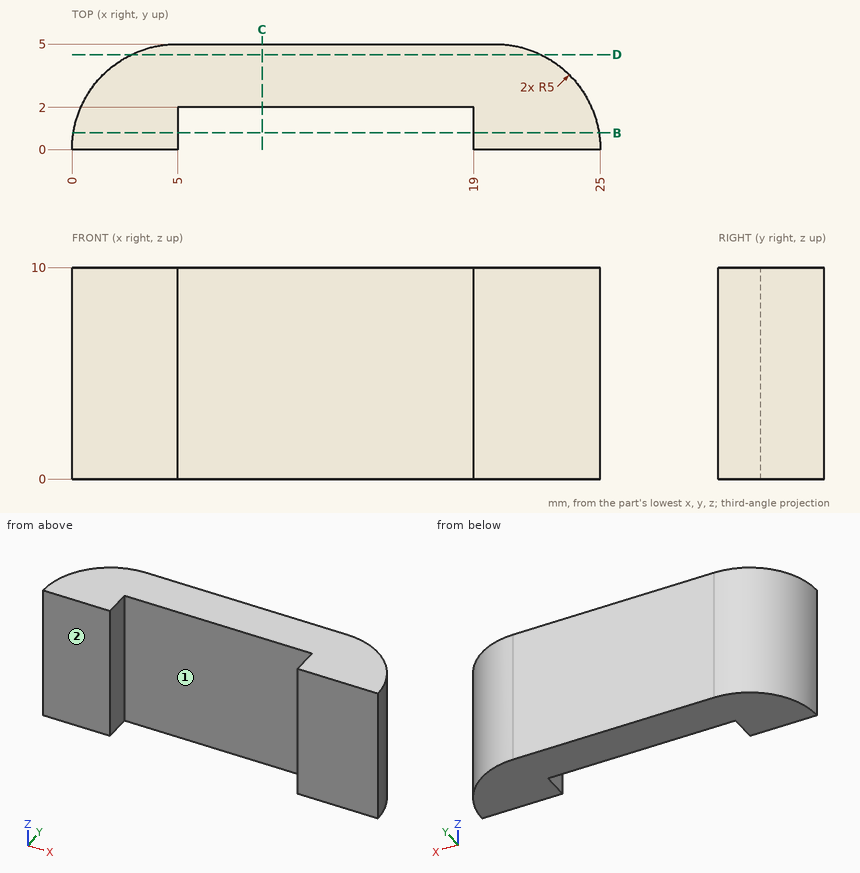
Drawing for the job (mm, zero at the part's lowest x, y, z). A direction names the side the tool comes from. Round coordinates to 2 decimals unless told otherwise and drop trailing zeros. Loops run counter-clockwise (first coordinate to the right, second up) from the corner with the lowest first, then second, coordinate; pieces in that order, holes last.
1. Band-saw the part on B-B, the plane y = 0.8. List the corners of the cut face in (x, z).
Check values:
outline: (0.06, 0) - (5, 0) - (5, 10) - (0.06, 10) - close; (19, 0) - (24.94, 0) - (24.94, 10) - (19, 10) - close
2. Band-saw the part on D-D, the plane y = 4.5. List the corners of the cut face in (x, z).
Check values:
outline: (2.82, 0) - (22.18, 0) - (22.18, 10) - (2.82, 10) - close
3. Tool access for the marked faces 1 and 2: list every direction of +Z, -Z, +X, -X, +Y, -Y with a clear straight run to the whole face (end or side of a thin tool).
Check values:
face 1: +Z, -Z, -Y
face 2: +Z, -Z, +X, -X, -Y
4. Wall check: probe 1 along Y at (x, z) = (17, 2.5); probe 2 along X at (y, z) = (1.9, 1.25) (3 decimals); probe 3 along X at (y, z) = (3, 5.75). Give the ranges that are in metal, low to high.
Check values:
probe 1: y = 2 to 5
probe 2: x = 0.375 to 5, 19 to 24.625
probe 3: x = 1 to 24
5. Drop flat-ended pins along their axis: P1, Ø1, axis at y = 1, z = 7, coming from the +X side (3 decimals); P2, Ø1, axis at x = 21.5, z = 5, coming from the +Y side; P3, Ø3, axis at x = 13.5, z = 4, coming from the -Y side. Give the stop position or say it passes through.
Check values:
P1: stops at x = 24.975
P2: stops at y = 4.9
P3: stops at y = 2
6. Band-saw the part on C-C, the plane x = 9. List the corners of the cut face in (y, z), and give its area (3 significant figures).
Check values:
outline: (2, 0) - (5, 0) - (5, 10) - (2, 10) - close
area: 30.0 mm2
